Input: part model. Units: mm. Frame: model coordinates. A direction names the side the tool comes from. Coordinates: 2 decimals unless noted, no trailing zeros. Write each loop counter-clockwise with the first axis right and the second up, starting at its lowest first coordinate (ties: lowest second). Pieces come first, ordered by that corner, then holes. Notation, with made-up numbers: M 56.5,-32 L 87.5,-32 A21 ccw 87.5,-8 Z; hole C -18.75,49.25 d2. An arc over 180 degrees is marked long. Use one line per item in the form item = value.
from build123d import *

# Parameters (mm, degrees)
SKETCH1_W           = 38.1
SKETCH1_H           = 31.75
SKETCH1_W_2         = 13
SKETCH1_H_2         = 19.4
BOSS_EXTRUDE1_DEPTH = 2.54
SKETCH2_W           = 38.1
SKETCH2_H           = 31.75
SKETCH2_W_2         = 33.02
SKETCH2_H_2         = 26.67
BOSS_EXTRUDE2_DEPTH = 22.225
SKETCH3_R           = 1.7145
BOSS_EXTRUDE3_DEPTH = 3.175
CUT_EXTRUDE1_REACH  = 61.791


with BuildPart() as part:
    # Sketch1 → Boss-Extrude1 (new body)
    with BuildSketch(Plane.XY):
        with Locations((19.05, 15.875)):
            Rectangle(SKETCH1_W, SKETCH1_H)
        with Locations((10.533333333, 15.875)):
            Rectangle(SKETCH1_W_2, SKETCH1_H_2, mode=Mode.SUBTRACT)
        with Locations((27.566666667, 15.875)):
            Rectangle(SKETCH1_W_2, SKETCH1_H_2, mode=Mode.SUBTRACT)
    extrude(amount=BOSS_EXTRUDE1_DEPTH)

    # Sketch2 → Boss-Extrude2 (add)
    with BuildSketch(Plane(origin=(0, 0, 0), x_dir=(-1, 0, 0), z_dir=(0, 0, -1))):
        with Locations((-19.05, 15.875)):
            Rectangle(SKETCH2_W, SKETCH2_H)
        with Locations((-19.05, 15.875)):
            Rectangle(SKETCH2_W_2, SKETCH2_H_2, mode=Mode.SUBTRACT)
    extrude(amount=BOSS_EXTRUDE2_DEPTH)

    # Sketch3 → Boss-Extrude3 (add)
    # profile 1 of 2: a face of its own
    with BuildSketch(Plane(origin=(0, 0, -22.225), x_dir=(-1, 0, 0), z_dir=(0, 0, -1))):
        with BuildLine():
            Line((-41.91, 19.4945), (-38.1, 19.4945))
            Line((-38.1, 19.4945), (-38.1, 12.2555))
            Line((-38.1, 12.2555), (-41.91, 12.2555))
            ThreePointArc((-41.91, 12.2555), (-45.5295, 15.875), (-41.91, 19.4945))
        make_face()
        with Locations((-41.91, 15.875)):
            Circle(SKETCH3_R, mode=Mode.SUBTRACT)
    # profile 2 of 2: a face of its own
    with BuildSketch(Plane(origin=(0, 0, -22.225), x_dir=(-1, 0, 0), z_dir=(0, 0, -1))):
        with BuildLine():
            Line((3.81, 12.2555), (0, 12.2555))
            Line((0, 12.2555), (0, 19.4945))
            Line((0, 19.4945), (3.81, 19.4945))
            ThreePointArc((3.81, 19.4945), (7.4295, 15.875), (3.81, 12.2555))
        make_face()
        with Locations((3.81, 15.875)):
            Circle(SKETCH3_R, mode=Mode.SUBTRACT)
    extrude(amount=-BOSS_EXTRUDE3_DEPTH)

    # Sketch4 → Cut-Extrude1 (cut, up to next)
    with BuildSketch(Plane.XZ, mode=Mode.PRIVATE) as cut_extrude1_sk1:
        with BuildLine():
            Line((22.225, -19.05), (22.225, -22.225))
            Line((22.225, -22.225), (15.875, -22.225))
            Line((15.875, -22.225), (15.875, -19.05))
            ThreePointArc((15.875, -19.05), (19.05, -15.875), (22.225, -19.05))
        make_face()
    cut_extrude1_tool1 = extrude(cut_extrude1_sk1.sketch, amount=-CUT_EXTRUDE1_REACH, mode=Mode.PRIVATE) & part.part
    add(cut_extrude1_tool1.solids().sort_by_distance((19.05, 0, -19.346386))[0], mode=Mode.SUBTRACT)


solid = part.part
(1) First-contact query: pin 1 Ø2 at (y, z) = (9.5, -3) entering from +X; pin 2 Ø6 at (x, y) = (42.5, 15.5) entering from +Z; pin 3 Ø1.6 at (x, z) = (40, -21) entering from -Y. Flat tips, straight axial feed; report the tip coordinate or a pass-through.
Computed:
pin_1 = 38.1
pin_2 = -19.05
pin_3 = 12.26
(2) Set-up query: faces 5 (the flat face through (-2, 12.256, -21)), 6 (the flat face through (19, 17, 0)), 7 (the flat face through (10, 6.175, 1)). Return all of +Z, -Z, +X, -X, +Y, -Y with unobstructed straight access to the full face (end or side cutting, diameter ignored); none if empty.
Computed:
face_5 = +Z, -Z, -X, -Y
face_6 = -Z
face_7 = +Z, -Z
(3) Section query D-D on y = 4. Return the cut outline in (x, z) (3 decimals), plus the area to 3 significant figures.
Computed:
outline = M 0,-22.225 L 2.54,-22.225 L 2.54,0 L 35.56,0 L 35.56,-22.225 L 38.1,-22.225 L 38.1,2.54 L 0,2.54 Z
area = 210 mm^2
(4) Line query: probe 1 along X at (y, z) = (23, 0.75); probe 2 along X at (y, z) = (22.5, -2); probe 3 along Y at (x, z) = (41.91, -21.2). Output: solid intervals per line, ascending.
Computed:
probe_1 = 0 to 4.03, 17.03 to 21.07, 34.07 to 38.1
probe_2 = 0 to 2.54, 35.56 to 38.1
probe_3 = 12.26 to 14.16, 17.59 to 19.49
(5) Section query C-C on x = 19.05. Return the cut outline in (y, z) (3 decimals).
Computed:
outline = M 0,-15.875 L 2.54,-15.875 L 2.54,0 L 29.21,0 L 29.21,-22.225 L 31.75,-22.225 L 31.75,2.54 L 0,2.54 Z
(6) Pull-direction query (X, two-part tool) for faces 1 (the flat face through (27, 6.175, 1)), 2 (the flat face through (19, 0, -10)), 3 (the cylindrical face through (45.53, 15.8, -20.66)), 4 (the flat face through (17.033, 16, 1)); classes: pulls with the +X half, pulls with the -X half, needs draft (parallel to the pull), parting line crosses it, or undercut.
Computed:
face_1 = undercut
face_2 = needs draft
face_3 = pulls with the +X half
face_4 = undercut
(7) Section query A-A on z = -11.5. Return the cut outline in (x, y), plus the area to 3 significant figures.
Computed:
outline = M 0,0 L 38.1,0 L 38.1,31.75 L 0,31.75 Z; hole M 2.54,2.54 L 35.56,2.54 L 35.56,29.21 L 2.54,29.21 Z
area = 329 mm^2
(8) Section query B-B on y = 23. Return the cut outline in (x, z) (3 decimals).
Computed:
outline = M 0,-22.225 L 2.54,-22.225 L 2.54,0 L 4.033,0 L 4.033,2.54 L 0,2.54 Z; M 17.033,0 L 21.067,0 L 21.067,2.54 L 17.033,2.54 Z; M 34.067,0 L 35.56,0 L 35.56,-22.225 L 38.1,-22.225 L 38.1,2.54 L 34.067,2.54 Z
